from build123d import *

# Parameters (mm, degrees)
F0_W     = 6
F0_H     = 3.6
F1_DEPTH = 25
F2_SIZE2 = 0.75
F2_SIZE  = 2


with BuildPart() as f1:
    # F0 (on Front) → F1 (new body)
    with BuildSketch(Plane.XZ):
        with Locations((-1.260776, -2.620722)):
            Rectangle(F0_W, F0_H)
    extrude(amount=F1_DEPTH)

    # F2
    f2_edges = [f1.edges().sort_by_distance(p)[0] for p in [
        (-1.260776, -25, -0.820722),
        (-1.260776, -25, -4.420722),
    ]]
    chamfer(f2_edges, length=F2_SIZE, length2=F2_SIZE2)


solid = f1.part
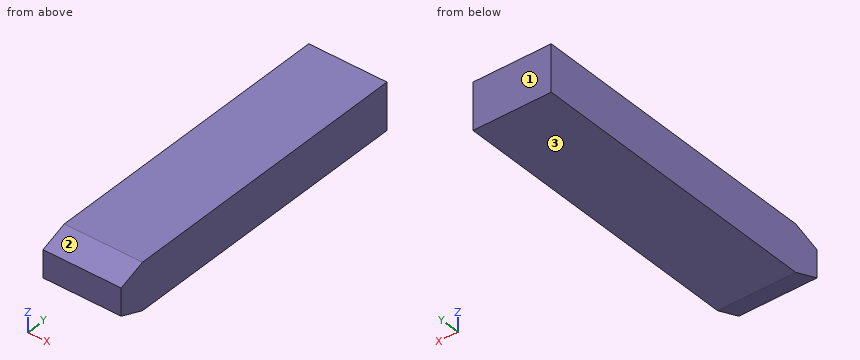
The listing builds one solid part. Answer for the finished solid, in the listing's coordinates (mm). Face numbers are marked on the shaded views. Give positions to 0.01 mm unless a question says otherwise; leave off trailing zeros. Loops run counter-clockwise (first coordinate to the right, second up) from the corner with the lowest first, then second, coordinate; pieces in that order, holes last. Notation, with made-up numbers: M 73.5,33.5 L 101.5,33.5 A24 cw 101.5,46.5 Z; hole C -18,29.5 d4. An arc over 180 degrees is marked long. Answer as CSV lines item,"result".
Item 1: The mould has two halves that part along Y. Classify the marked faces 1, 2 and 3: released by +Y, released by -Y, zero draft, split by the parting line, or undercut.
Values follow:
face 1,"released by +Y"
face 2,"released by -Y"
face 3,"zero draft"
Item 2: The part is cut by section B-B (z = -1.2). Give the vertices of the cut face in (x, y), and give its area (3 significant figures).
Values follow:
outline,"M -4.26,-24.01 L 1.74,-24.01 L 1.74,0 L -4.26,0 Z"
area,"144 mm^2"
Item 3: The part is cut by section A-A (x = -2.75). Give the vertices of the cut face in (y, z).
Values follow:
outline,"M -25,-3.67 L -23,-4.42 L 0,-4.42 L 0,-0.82 L -23,-0.82 L -25,-1.57 Z"
